Work out the finished part from the listing and answer in its coordinate system (mm). Face numbers are marked on the shaded views. Give positions to 0.01 mm unless a question says otherwise; leave off trailing zeros. Loops run counter-clockwise (first coordinate to the right, second up) from the corner with the lowest first, then second, coordinate; pieces in that order, holes last. Notation, with made-up numbers: (-28, 67) - (29, 67) arc R13 ccw to (29, 85) - close; hole circle Ø6 at (33.25, -30). An arc over 180 degrees is marked (long way). One line per question, with ' | ' between items. Start each with the question number.
1. Section C-C (x = 37) is taken. Determine the outline of the cut face in (y, z), plus the area to 3 significant figures.
2. Each of these flat-tipped pins is pushed along its axis until it touches: pin 1 (2 mm diameter, centred on x = 23, z = 0.5, fed in from +Y); pin 2 (1 mm diameter, centred on x = 16.5, z = -1, fed in from -Y). Where does it stop, or does it pass through?
3. For a pull along X with two mould halves and no side action, classify the marked faces 1, 2, 3 and 4 as released by +X, released by -X, zero draft, split by the parting line, or undercut.
4. Find the intervals of material crossed by line 1 (Z direction, x = 23.5, y = -1.05); line 2 (Z direction, x = 26.5, y = -0.1), in increasing order.
from build123d import *

# Parameters (mm, degrees)
SKETCH2_W     = 8
SKETCH2_H     = 2
SKETCH2_W_2   = 24
FILLET1_R     = 0.2
CHAMFER1_SIZE = 0.3


with BuildPart() as part:
    # Sketch2 → Revolve1 (revolve)
    with BuildSketch(Plane.XY, mode=Mode.PRIVATE) as revolve1_sk:
        with Locations((4, 1)):
            Rectangle(SKETCH2_W, SKETCH2_H)
        with Locations((14, 1)):
            Rectangle(SKETCH2_W, SKETCH2_H)
        Polygon((8, 2.25), (8, 2), (8, 0), (10, 0), (10, 2), (9, 2), (9, 2.25), align=None)
        with Locations((30, 1)):
            Rectangle(SKETCH2_W_2, SKETCH2_H)
        with Locations((46, 1)):
            Rectangle(SKETCH2_W, SKETCH2_H)
        Polygon((50, 2), (50, 0), (58, 0), (58, 2), (58, 2.25), (57, 2.25), (57, 2), align=None)
        with Locations((62, 1)):
            Rectangle(SKETCH2_W, SKETCH2_H)
    revolve(revolve1_sk.sketch.rotate(Axis((0, 0, 0), (1, 0, 0)), 90), axis=Axis((0, 0, 0), (1, 0, 0)))

    # Fillet1
    fillet1_edges = [part.edges().sort_by_distance(p)[0] for p in [
        (8, 0, -2),
        (9, 0, -2),
        (57, 0, -2),
        (58, 0, -2),
    ]]
    fillet(fillet1_edges, radius=FILLET1_R)

    # Chamfer1
    chamfer1_edges = [part.edges().sort_by_distance(p)[0] for p in [
        (0, 0, -2),
        (66, 0, -2),
    ]]
    chamfer(chamfer1_edges, length=CHAMFER1_SIZE)


solid = part.part
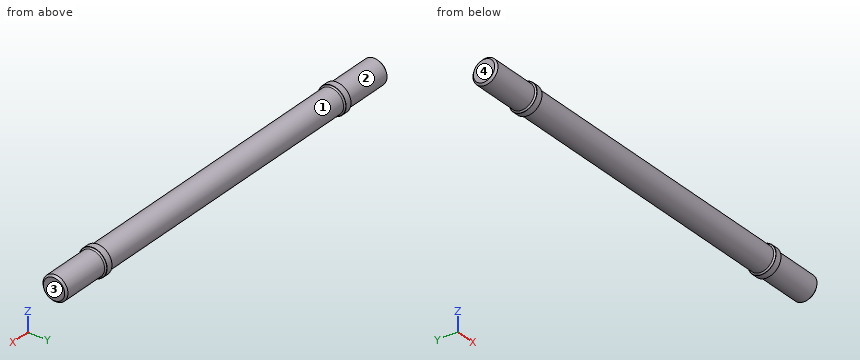
Conclusion:
1) outline: circle Ø4 at (0, 0) | area: 12.6 mm²
2) pin 1: y = 2 | pin 2: y = -1.94
3) face 1: undercut | face 2: zero draft | face 3: released by +X | face 4: released by -X
4) line 1: -1.7 to 1.7 | line 2: -2 to 2
